Autodesk Inventor part; units mm, degrees
ref_plane "YZ Plane" through (0, 0, 0) normal (1, 0, 0) x (0, 1, 0)
ref_plane "XZ Plane" through (0, 0, 0) normal (0, 1, 0) x (-1, 0, 0)
ref_plane "XY Plane" through (0, 0, 0) normal (0, 0, 1) x (1, 0, 0)
sketch "Schizzo1" plane through (0, 0, 0) normal (1, 0, 0) x (0, 1, 0)
  line L0 (-35, -40) -> (35, -40)
  line L1 (40, -35) -> (40, 35)
  line L2 (35, 40) -> (-35, 40)
  line L3 (-40, 35) -> (-40, -35)
  line L4 (-40, -40) -> (40, 40) construction
  line L5 (40, -40) -> (-40, 40) construction
  arc A0 (40, 35) -> (35, 40) centre (35, 35) ccw
  arc A1 (35, -40) -> (40, -35) centre (35, -35) ccw
  arc A2 (-35, 40) -> (-40, 35) centre (-35, 35) ccw
  arc A3 (-40, -35) -> (-35, -40) centre (-35, -35) ccw
  circle A4 centre (0, 0) radius 22.5
  dimension "d4" = 45
extrude "Estrusione1" add sketch "Schizzo1" along normal mid plane 2
sketch "Schizzo2" plane through (1, 0, 0) normal (1, 0, 0) x (0, 0, -1)
  circle A0 centre (0, 0) radius 30
  circle A1 centre (0, 30) radius 6.0177
  circle A2 centre (-25.9808, 15) radius 6.0177
  circle A3 centre (-25.9808, -15) radius 6.0177
  circle A4 centre (0, -30) radius 6.0177
  circle A5 centre (25.9808, -15) radius 6.0177
  circle A6 centre (25.9808, 15) radius 6.0177
  circle A7 centre (-25.9808, 15) radius 5.5175
  circle A8 centre (-25.9808, 15) radius 5.0175
  circle A9 centre (-25.9808, 15) radius 4.5175
  circle A10 centre (-25.9808, 15) radius 4.0175
  circle A11 centre (-25.9808, 15) radius 3.5175
  circle A12 centre (0, -30) radius 6.0177
  circle A13 centre (-25.9808, -15) radius 3.5175
  circle A14 centre (-25.9808, -15) radius 4.0175
  circle A15 centre (-25.9808, -15) radius 4.5175
  circle A16 centre (-25.9808, -15) radius 5.0175
  circle A17 centre (-25.9808, -15) radius 5.5175
  circle A18 centre (25.9808, -15) radius 6.0177
  circle A19 centre (0, -30) radius 3.5175
  circle A20 centre (0, -30) radius 4.0175
  circle A21 centre (0, -30) radius 4.5175
  circle A22 centre (0, -30) radius 5.0175
  circle A23 centre (0, -30) radius 5.5175
  circle A24 centre (25.9808, 15) radius 6.0177
  circle A25 centre (25.9808, -15) radius 3.5175
  circle A26 centre (25.9808, -15) radius 4.0175
  circle A27 centre (25.9808, -15) radius 4.5175
  circle A28 centre (25.9808, -15) radius 5.0175
  circle A29 centre (25.9808, -15) radius 5.5175
  circle A30 centre (0, 30) radius 6.0177
  circle A31 centre (25.9808, 15) radius 3.5175
  circle A32 centre (25.9808, 15) radius 4.0175
  circle A33 centre (25.9808, 15) radius 4.5175
  circle A34 centre (25.9808, 15) radius 5.0175
  circle A35 centre (25.9808, 15) radius 5.5175
  circle A36 centre (-25.9808, 15) radius 6.0177
  circle A37 centre (0, 30) radius 3.5175
  circle A38 centre (0, 30) radius 4.0175
  circle A39 centre (0, 30) radius 4.5175
  circle A40 centre (0, 30) radius 5.0175
  circle A41 centre (0, 30) radius 5.5175
  circle A42 centre (-25.9808, 15) radius 3.0175
  dimension "d7" = 60
  dimension "d10" = 360
  dimension "d13" = 11.035
  dimension "d14" = 10.035
  dimension "d15" = 9.035
  dimension "d16" = 8.035
  dimension "d17" = 7.035
  dimension "d20" = 360
  dimension "d24" = 6.035
extrude "Estrusione2" cut sketch "Schizzo2" against normal blind 0.5 contours A6 A0 A35 | A0 A35 A6 | A5 A0 A29 | A0 A29 A5 | A35 A0 A34 | A0 A34 A35 | A29 A0 A28 | A0 A28 A29 | A1 A0 A41 | A0 A41 A1 | A28 A0 A27 | A0 A27 A28 | A4 A0 A23 | A0 A23 A4 | A23 A0 A22 | A0 A22 A23 | A2 A0 A7 | A0 A7 A2 | A22 A0 A21 | A0 A21 A22 | A3 A0 A17 | A0 A17 A3 | A7 A0 A8 | A0 A8 A7 | A21 A0 A20 | A0 A20 A21 | A17 A0 A16 | A0 A16 A17 | A8 A0 A9 | A0 A9 A8 | A16 A0 A15 | A0 A15 A16 | A9 A0 A10 | A0 A10 A9 | A15 A0 A14 | A0 A14 A15 | A10 A0 A11 | A0 A11 A10 | A14 A0 A13 | A0 A13 A14 | A11 A0 A42 | A0 A42 A11
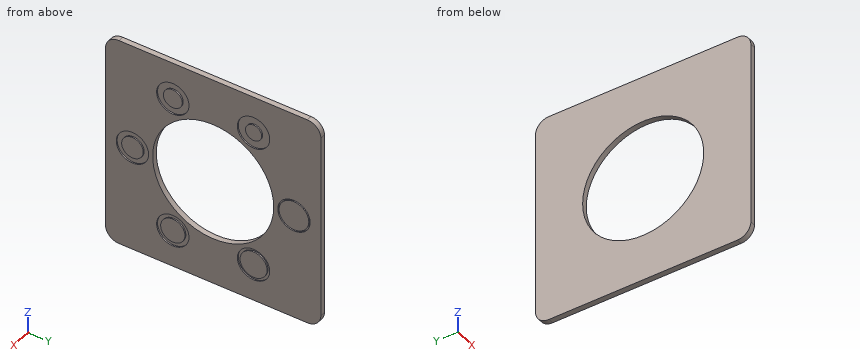
Verification items for the finished model (mm, model axes). Coordinates: 2 decimals unless noted, no trailing zeros. Write each loop counter-clockwise with the first axis right and the second up, starting at its lowest first coordinate (ties: lowest second). Pieces come first, ordered by that corner, then holes. Notation, with made-up numbers: (63.25, 8) -> (75.25, 8) arc R35 cw to (75.25, 45) -> close; hole circle Ø4 at (-40, 1). An arc over 180 degrees is marked (long way). One line per item, written item: value. Start each with the question number.
Q1. Cross-section at C-C on z = 0. Enter the section's corners in (x, y), and give its area (3 significant figures).
Q2. Cross-section at D-D on y = 16. Enter the section's corners in (x, z).
Q3. Cross-section at A-A on y = 0. Enter the section's corners in (x, z).
Q4. Thickness scan on L1, parallel to Z at x = -0.45, y = 0; L2, parallel to Z at x = 0.7, y = -9.5; L3, parallel to Z at x = 0.75, y = 27. Record the ranges inside material, lowest first. Write a range as from..to.
Q5. Cross-section at B-B on x = -0.2. Enter the section's corners in (y, z), and give its area (3 significant figures).
Checked values:
1. outline: (-1, -40) -> (1, -40) -> (1, -36.02) -> (0.5, -36.02) -> (0.5, -34.02) -> (1, -34.02) -> (1, -25.98) -> (0.5, -25.98) -> (0.5, -23.98) -> (1, -23.98) -> (1, -22.5) -> (-1, -22.5) -> close; (-1, 22.5) -> (1, 22.5) -> (1, 23.98) -> (0.5, 23.98) -> (0.5, 24.48) -> (1, 24.48) -> (1, 35.52) -> (0.5, 35.52) -> (0.5, 36.02) -> (1, 36.02) -> (1, 40) -> (-1, 40) -> close
1. area: 67.5 mm²
2. outline: (-1, -40) -> (1, -40) -> (1, -31.91) -> (0.5, -31.91) -> (0.5, -30.9) -> (1, -30.9) -> (1, -21.06) -> (0.5, -21.06) -> (0.5, -20.05) -> (1, -20.05) -> (1, -15.82) -> (-1, -15.82) -> close; (-1, 15.82) -> (1, 15.82) -> (1, 20.05) -> (0.5, 20.05) -> (0.5, 23.13) -> (1, 23.13) -> (1, 28.83) -> (0.5, 28.83) -> (0.5, 31.91) -> (1, 31.91) -> (1, 40) -> (-1, 40) -> close
3. outline: (-1, -40) -> (1, -40) -> (1, -22.5) -> (-1, -22.5) -> close; (-1, 22.5) -> (1, 22.5) -> (1, 40) -> (-1, 40) -> close
4. L1: z = -40..-22.5, 22.5..40
4. L2: z = -40..-28.42, -23.54..-20.4, 20.4..23.54, 28.42..40
4. L3: z = -40..-5.22, -4.63..4.63, 5.22..40
5. outline: (-40, -35) arc R5 ccw to (-35, -40) -> (35, -40) arc R5 ccw to (40, -35) -> (40, 35) arc R5 ccw to (35, 40) -> (-35, 40) arc R5 ccw to (-40, 35) -> close; hole circle Ø45 at (0, 0)
5. area: 4,790 mm²
